from build123d import *

# Parameters (mm, degrees)
F1_DEPTH = 25


with BuildPart() as f1:
    # F0 (on Top) → F1 (new body)
    with BuildSketch(Plane.XY):
        with BuildLine():
            Line((0, 0), (-20, 30))
            Line((-20, 30), (-30, 30))
            Line((-30, 30), (-44.90712, 13.333333))
            ThreePointArc((-44.90712, 13.333333), (-50, 0), (-44.90712, -13.333333))
            Line((-44.90712, -13.333333), (-30, -30))
            Line((-30, -30), (-17.320508, -30))
            ThreePointArc((-17.320508, -30), (0, -20), (17.320508, -30))
            Line((17.320508, -30), (30, -30))
            Line((30, -30), (30, 30))
            Line((30, 30), (20, 30))
            Line((20, 30), (0, 0))
        make_face()
    extrude(amount=F1_DEPTH)


solid = f1.part
Part model, mm, in its own coordinate system. A direction names the side the tool comes from. Round coordinates to 2 decimals unless told otherwise and drop trailing zeros. Loops run counter-clockwise (first coordinate to the right, second up) from the corner with the lowest first, then second, coordinate; pieces in that order, holes last. Notation, with made-up numbers: (-17, -5) - (10, -5) arc R30 cw to (10, 19) - close; hole circle Ø6 at (-26.5, -6). An arc over 180 degrees is marked (long way). Answer as a JSON object with one key per item and string values.
Item 1: Tool access for faces 1 (the face through (24, -30, 12)), 2 (the face through (-10, 15, 12)): list every direction of +Z, -Z, +X, -X, +Y, -Y with a clear straight run to the whole face (end or side of a thin tool).
Output:
{"face 1": "+Z, -Z, +X, -X, -Y", "face 2": "+Z, -Z, +Y"}
Item 2: Pull direction X, two halves, no side cores. Call faces 3 (the face through (-50, 0, 12)), 4 (the face through (10, 15, 12)), 5 (the face through (-11, 0, 25)), 6 (the face through (0, -20, 12)): pulls with the +X half, pulls with the -X half, needs draft (parallel to the pull), parting line crosses it, or undercut.
Output:
{"face 3": "pulls with the -X half", "face 4": "undercut", "face 5": "needs draft", "face 6": "undercut"}
Item 3: Band-saw the part on B-B on z = 14.5. List the corners of the cut face in (x, y), plus the area to 3 significant figures.
Output:
{"outline": "(-44.91, -13.33) - (-30, -30) - (-17.32, -30) arc R20 cw to (17.32, -30) - (30, -30) - (30, 30) - (20, 30) - (0, 0) - (-20, 30) - (-30, 30) - (-44.91, 13.33) arc R20 ccw to start", "area": "3,490 mm2"}
Item 4: Band-saw the part on A-A on y = -21.5. List the corners of the cut face in (x, z).
Output:
{"outline": "(-37.6, 0) - (-7.6, 0) - (-7.6, 25) - (-37.6, 25) - close; (7.6, 0) - (30, 0) - (30, 25) - (7.6, 25) - close"}
Item 5: Wall check: L1, parallel to X at y = 1, z = 11; L2, parallel to X at y = 8, z = 13; L3, parallel to X at y = -7.5, z = 4.75. Give the ranges that are in metal, low to high.
Output:
{"L1": "-49.97 to -0.67, 0.67 to 30", "L2": "-48.33 to -5.33, 5.33 to 30", "L3": "-48.54 to 30"}
Item 6: Pin check, flat tips, straight feed: pin 1 (4 mm diameter, centred on x = 9.5, z = 5, fed in from +Y); pin 2 (4 mm diameter, centred on x = 9.5, z = 4, fed in from -Y); pin 3 (1.5 mm diameter, centred on x = 5.5, z = 13.5, fed in from -Y). Stop position of each tip, or through.
Output:
{"pin 1": "y = 17.25", "pin 2": "y = -23.64", "pin 3": "y = -21"}
Item 7: Band-saw the part on C-C on y = 10.5. List the corners of the cut face in (x, z), plus the area to 3 significant figures.
Output:
{"outline": "(-47.02, 0) - (-7, 0) - (-7, 25) - (-47.02, 25) - close; (7, 0) - (30, 0) - (30, 25) - (7, 25) - close", "area": "1,580 mm2"}
Item 8: Band-saw the part on D-D on x = 19. List the corners of the cut face in (y, z), plus the area to 3 significant figures.
Output:
{"outline": "(-30, 0) - (28.5, 0) - (28.5, 25) - (-30, 25) - close", "area": "1,460 mm2"}
